The model under review builds one solid part; all positions refer to its coordinate system, in mm. A direction names the side the tool comes from. Coordinates: 2 decimals unless noted, no trailing zeros. Order: outer loops, then holes, each group sorted by start corner. A loop starts at its lowest first (then second) coordinate and runs counter-clockwise, first axis right, second up. Notation, with made-up numbers: (-21.75, 70) -> (9.25, 70) arc R30 cw to (9.25, 96) -> close; hole circle Ø7 at (85, 24). An arc over 180 degrees is marked (long way). Use one line per item in the form item = value. Start each with the question number.
(1) Insertion check: pin 1 Ø1.5 at (y, z) = (11.5, -0.5) entering from -X; pin 2 Ø2 at (x, z) = (1.5, 1.5) entering from -Y; pin 3 Ø1.5 at (x, z) = (10.5, -1) entering from +Y. Each pin has a flat end and moves straight along its axis. Give the tip position at first contact, or say it passes through.
(2) Wall thickness on line 1 along X through (y, z) = (0, -0.6); line 2 along Z through (x, y) = (31, -10): over which ranges is each line inside the solid? List them lowest first.
(3) Take a section at A-A (x = 0). State the section outline as (y, z) points (3 decimals), then the cut area to 4 significant figures.
(4) For faces 5 (the cylindrical face through (33.28, 40.13, 0.01)), 6 (the flat face through (24, 1, -1)), 7 (the cylindrical face through (-50.6, 12.6, 0)), list the 3-axis set-ups (+Z, -Z, +X, -X, +Y, -Y) from which the entire face can be reached by the end or side of a thin tool; tool diameter is ignored.
(5) Mouldability with a two-part tool opening along Y and no side actions: class faces 1 (the cylindrical face through (20.03, 6.31, -1.31)), 2 (the flat face through (1, 17, 2.125)), 3 (the cylindrical face through (-12.6, -50.6, 0)), 4 (the cylindrical face through (40.13, -33.28, 0.01)) as +Y half, -Y half, draft (parallel to the pull), parting line (faces both ways), or undercut.
```python
from build123d import *

# Parameters (mm, degrees)
ESQUISSE1_R                  = 57
EXTRUSION1_DEPTH             = 1
ENL_V_MAT_EXTRU_1_DEPTH      = 2
R_P_TITION_CIRCULAIRE1_COUNT = 28
ESQUISSE3_R                  = 21
EXTRUSION2_DEPTH             = 2.125
ESQUISSE4_R                  = 16
ENL_V_MAT_EXTRU_2_DEPTH      = 3.125
ENL_V_MAT_EXTRU_2_DEPTH_BACK = 3.125
CHANFREIN1_SIZE              = 0.5


with BuildPart() as part:
    # Esquisse1 → Extrusion1 (new body, symmetric)
    with BuildSketch(Plane.XY):
        Circle(ESQUISSE1_R)
    extrude(amount=EXTRUSION1_DEPTH, both=True)

    # Esquisse2 → Enlèv. mat.-Extru.1 (cut, symmetric)
    with BuildSketch(Plane.XY):
        with BuildLine():
            Line((-5.403559241, 56.743295177), (-3.276608177, 53.705694255))
            ThreePointArc((-3.276608177, 53.705694255), (1.065722501, 52.144583609), (3.98978287, 55.714285714))
            Line((3.98978287, 55.714285714), (4.071428571, 56.854405892))
            ThreePointArc((4.071428571, 56.854405892), (-0.668378207, 56.996081186), (-5.403559241, 56.743295177))
        make_face()
    enl_v_mat_extru_1 = extrude(amount=ENL_V_MAT_EXTRU_1_DEPTH, both=True, mode=Mode.SUBTRACT)

    # Répétition circulaire1: Enlèv. mat.-Extru.1 ×28 about axis
    r_p_tition_circulaire1_axis = Axis((0, 0, 0), (0, 0, 1))
    for i in range(1, R_P_TITION_CIRCULAIRE1_COUNT):
        add(enl_v_mat_extru_1.rotate(r_p_tition_circulaire1_axis, i * 360 / R_P_TITION_CIRCULAIRE1_COUNT), mode=Mode.SUBTRACT)

    # Esquisse3 → Extrusion2 (add, symmetric)
    with BuildSketch(Plane.XY):
        Circle(ESQUISSE3_R)
    extrude(amount=EXTRUSION2_DEPTH, both=True)

    # Esquisse4 → Enlèv. mat.-Extru.2 (cut, two sides)
    with BuildSketch(Plane.XY) as enl_v_mat_extru_2_sk:
        Circle(ESQUISSE4_R)
    extrude(amount=ENL_V_MAT_EXTRU_2_DEPTH, mode=Mode.SUBTRACT)
    extrude(enl_v_mat_extru_2_sk.sketch, amount=-ENL_V_MAT_EXTRU_2_DEPTH_BACK, mode=Mode.SUBTRACT)

    # Chanfrein1
    chanfrein1_edges = [part.edges().sort_by_distance(p)[0] for p in [
        (-21, 0, -2.125),
        (-21, 0, 2.125),
        (-16, 0, -2.125),
        (-16, 0, 2.125),
    ]]
    chamfer(chanfrein1_edges, length=CHANFREIN1_SIZE)


solid = part.part
```
Findings:
q1.pin_1 = -50.98
q1.pin_2 = -52.77
q1.pin_3 = 51.65
q2.line_1 = -52 to -16, 16 to 52
q2.line_2 = -1 to 1
q3.outline = (-52, -1) -> (-21, -1) -> (-21, -1.625) -> (-20.5, -2.125) -> (-16.5, -2.125) -> (-16, -1.625) -> (-16, 1.625) -> (-16.5, 2.125) -> (-20.5, 2.125) -> (-21, 1.625) -> (-21, 1) -> (-52, 1) -> close; (16, -1.625) -> (16.5, -2.125) -> (20.5, -2.125) -> (21, -1.625) -> (21, -1) -> (52, -1) -> (52, 1) -> (21, 1) -> (21, 1.625) -> (20.5, 2.125) -> (16.5, 2.125) -> (16, 1.625) -> close
q3.area = 165.5 mm²
q4.face_5 = +Z, -Z
q4.face_6 = -Z
q4.face_7 = +Z, -Z, -X
q5.face_1 = parting line
q5.face_2 = draft
q5.face_3 = -Y half
q5.face_4 = undercut
